The figure shows three views and two pictorial views of one solid part (mm, origin at its lowest corner). Answer the questions. A direction names the side the tool comes from. Give positions to 0.01 mm unless a question says otherwise; leave off trailing zeros. Write each loop counter-clockwise with the first axis right and the second up, starting at its lowest first coordinate (ties: lowest second). Pieces come first, ordered by that corner, then holes. Notation, with made-up numbers: (81.25, -23.75) -> (98.25, -23.75) arc R36 cw to (98.25, 12.25) -> close; hole circle Ø1 at (-8.75, 5). An arc over 180 degrees is marked (long way). Write each question's results on one line, items separated by ' | '. Start each with the question number.
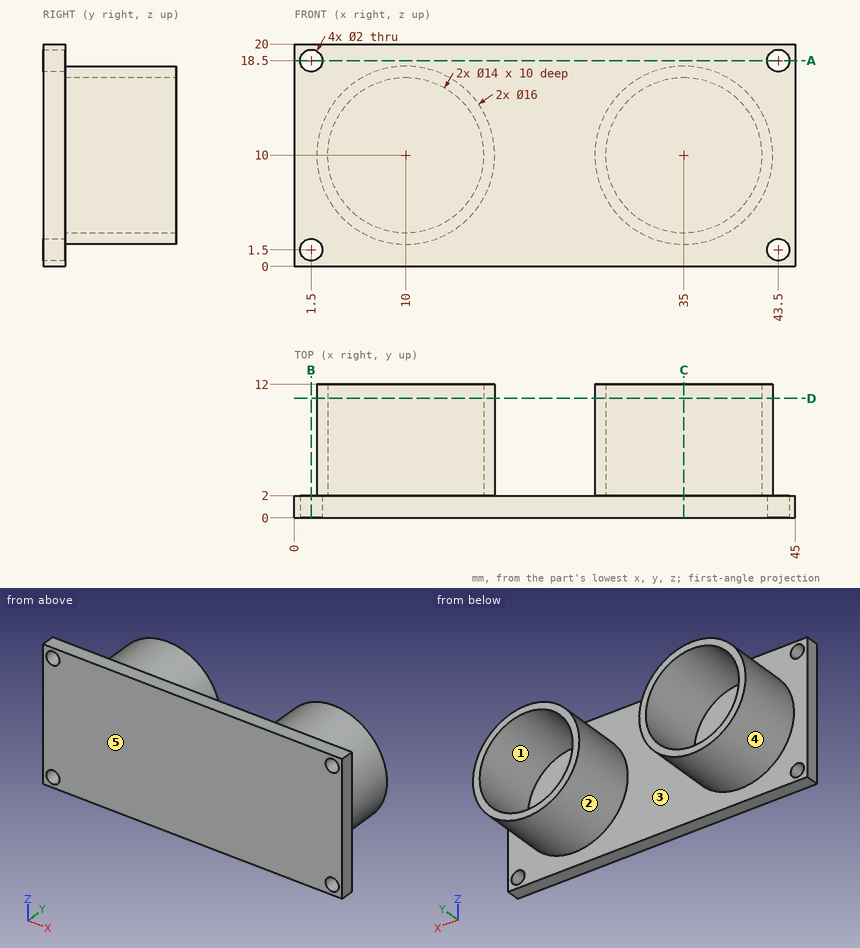
1. Each of these flat-tipped pins is pushed along its axis until it touches: pin 1 Ø4 at (y, z) = (8.5, 18) entering from +X; pin 2 Ø5 at (x, y) = (10.5, 7.5) entering from +Z; pin 3 Ø3 at (x, z) = (43.5, 1.5) entering from +Y. Where does it stop, or does it pass through?
2. Section A-A (z = 18.5) is taken. Write down the section's boundary in (x, y).
3. The mould has two halves that part along Z. Classify the marked faces 1, 2 and 3: pulls with the +Z half, pulls with the -Z half, needs draft (parallel to the pull), parting line crosses it, or undercut.
4. Consider probe 1 along X at (y, z) = (1.25, 18.5); probe 2 along Z at (x, y) = (43.5, 1.2); probe 3 along X at (y, z) = (2.5, 9.75). Determine where each line is inside the solid, lowest interval first. Write a range as [from, to].
5. A tool of negligible diameter and unlimited length cuts with its end or side. For the marked faces 4 and 5, from which of +Z, -Z, +X, -X, +Y, -Y can it reach the whole face along a straight path? Write none if from no direction.
6. Section C-C (x = 35) is taken. Write down the section's boundary in (y, z).
7. Section B-B (x = 1.5) is taken. Write down the section's boundary in (y, z), then the cut area to 3 significant figures.
8. Section D-D (y = 10.75) is taken. Write down the section's boundary in (x, z), then the cut area to 3 significant figures.
Results:
1) pin 1: stops at x = 40.29 | pin 2: stops at z = 18 | pin 3: stops at y = 2
2) outline: (0, 0) -> (0.5, 0) -> (0.5, 2) -> (0, 2) -> close; (2.5, 0) -> (42.5, 0) -> (42.5, 2) -> (2.5, 2) -> close; (44.5, 0) -> (45, 0) -> (45, 2) -> (44.5, 2) -> close
3) face 1: undercut | face 2: parting line crosses it | face 3: needs draft
4) probe 1: x = [0, 0.5], [2.5, 42.5], [44.5, 45] | probe 2: z = [0, 0.5], [2.5, 17.5], [19.5, 20] | probe 3: x = [2, 3], [17, 18], [27, 28], [42, 43]
5) face 4: +Y | face 5: +Z, -Z, +X, -X, -Y
6) outline: (0, 0) -> (2, 0) -> (2, 2) -> (12, 2) -> (12, 3) -> (2, 3) -> (2, 17) -> (12, 17) -> (12, 18) -> (2, 18) -> (2, 20) -> (0, 20) -> close
7) outline: (0, 0) -> (2, 0) -> (2, 0.5) -> (0, 0.5) -> close; (0, 2.5) -> (2, 2.5) -> (2, 17.5) -> (0, 17.5) -> close; (0, 19.5) -> (2, 19.5) -> (2, 20) -> (0, 20) -> close | area: 32.0 mm²
8) outline: circle Ø16 at (10, 10); circle Ø16 at (35, 10); hole circle Ø14 at (10, 10); hole circle Ø14 at (35, 10) | area: 94.2 mm²
